Part print with two shaded views. Sizes in mm from the minimum x, y, z corner. Coordinates: 2 decimals unless noted, no trailing zeros. Write each loop counter-clockwise with the first axis right and the second up, starting at its lowest first coordinate (ties: lowest second). Pieces come first, ordered by that corner, then holes. Notation, with made-up numbers: (10, 47.5) - (57, 47.5) arc R22 cw to (57, 61.5) - close; hole circle Ø7 at (60, 22.5). An arc over 180 degrees is marked (long way). Answer in a Markdown table with one row per item. Add a question column.
Q1. Pin check, flat tips, straight feed: pin 1 (6.5 mm diameter, centred on x = 48.31, z = 13.64, fed in from +Y); pin 2 (1 mm diameter, centred on y = 2.5, z = 34, fed in from +X); pin 3 (5 mm diameter, centred on x = 60.5, y = 1.5, fed in from +Z); pin 4 (3 mm diameter, centred on x = 119, z = 65, fed in from -Y). Stop position of each tip, or through.
Q2. Band-saw the part on D-D (x = 11). List the corners of the cut face in (y, z).
Q3. Band-saw the part on A-A (z = 65). List the corners of the cut face in (x, y), and give its area (3 significant figures).
Q4. Drill centre lines: line 1 along Z through (x, y) = (48, 4.75); line 2 along X through (y, z) = (0.75, 98) (1 decimal); line 3 along Y through (x, z) = (96, 77). Where is each one in solid material? Low to high. Write a range as from..to.
Q5. Band-saw the part on B-B (x = 65). List the corners of the cut face in (y, z).
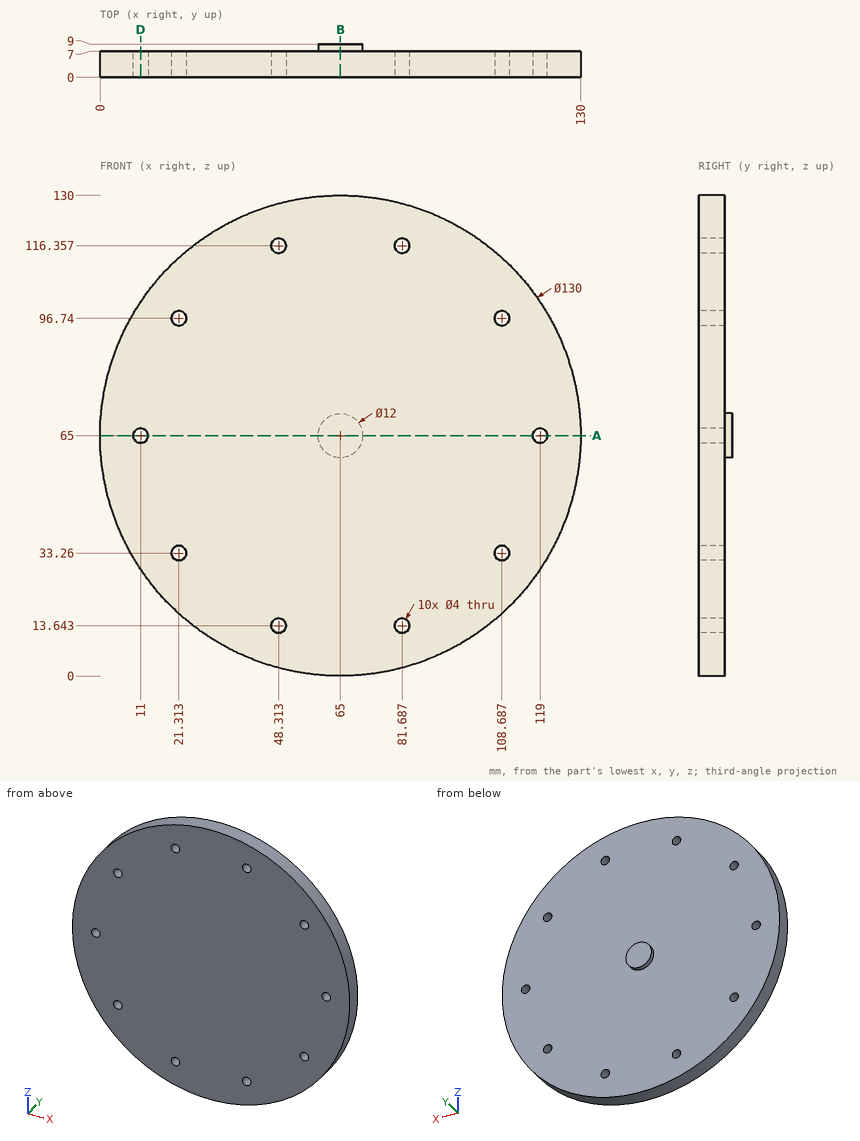
Checked values:
| question | item | result |
|---|---|---|
| 1 | pin 1 | stops at y = 7 |
| 1 | pin 2 | stops at x = 122.4 |
| 1 | pin 3 | stops at z = 129.97 |
| 1 | pin 4 | passes through |
| 2 | outline | (0, 28.82) - (7, 28.82) - (7, 63) - (0, 63) - close; (0, 67) - (7, 67) - (7, 101.18) - (0, 101.18) - close |
| 3 | outline | (0, 0) - (9, 0) - (9, 7) - (0, 7) - close; (13, 0) - (117, 0) - (117, 7) - (71, 7) - (71, 9) - (59, 9) - (59, 7) - (13, 7) - close; (121, 0) - (130, 0) - (130, 7) - (121, 7) - close |
| 3 | area | 878 mm² |
| 4 | line 1 | z = 2.26..11.67, 15.62..114.38, 118.33..127.74 |
| 4 | line 2 | x = 9..19.8, 22.9..107.1, 110.2..121 |
| 4 | line 3 | y = 0..7 |
| 5 | outline | (0, 0) - (7, 0) - (7, 59) - (9, 59) - (9, 71) - (7, 71) - (7, 130) - (0, 130) - close |
